from build123d import *

# Parameters (mm, degrees)
SKETCH_1_W          = 37.6
SKETCH_1_H          = 21
EXTRUDE_1_DEPTH     = 2
SKETCH_2_W          = 2.3
SKETCH_2_H          = 5.5
CUT_EXTRUDE_1_DEPTH = 22.626141588
SKETCH_4_W          = 13
SKETCH_4_H          = 10
EXTRUDE_2_DEPTH     = 2
EXTRUDE_4_DEPTH     = 10
SKETCH_6_R          = 6
CUT_EXTRUDE_2_DEPTH = 26.153329799
FILLET_1_R          = 2
FILLET_2_R          = 1


with BuildPart() as part:
    # 草图1 → 凸台-拉伸1 (new body)
    with BuildSketch(Plane.XY):
        Rectangle(SKETCH_1_W, SKETCH_1_H)
    extrude(amount=EXTRUDE_1_DEPTH)

    # 草图2 → 切除-拉伸1 (cut, through all)
    with BuildSketch(Plane.XY.offset(2)):
        with Locations((-17.65, 7.75)):
            Rectangle(SKETCH_2_W, SKETCH_2_H)
        with Locations((17.65, 7.75)):
            Rectangle(SKETCH_2_W, SKETCH_2_H)
        with Locations((-17.65, -7.75)):
            Rectangle(SKETCH_2_W, SKETCH_2_H)
        with Locations((17.65, -7.75)):
            Rectangle(SKETCH_2_W, SKETCH_2_H)
    extrude(amount=-CUT_EXTRUDE_1_DEPTH, mode=Mode.SUBTRACT)

    # 草图4 → 凸台-拉伸2 (add)
    with BuildSketch(Plane.ZY.offset(18.8)):
        with Locations((6.5, 0)):
            Rectangle(SKETCH_4_W, SKETCH_4_H)
    extrude_2 = extrude(amount=-EXTRUDE_2_DEPTH)

    # 草图5 → 凸台-拉伸4 (add)
    with BuildSketch(Plane(origin=(0, 5, 0), x_dir=(1, 0, 0), z_dir=(0, 1, 0))):
        Polygon((-8.740415593, -6.037395696), (-16.8, -10.690598923), (-16.8, -13), (-7.740415593, -7.769446504), align=None)
    extrude_4 = extrude(amount=-EXTRUDE_4_DEPTH)

    # 草图6 → 切除-拉伸2 (cut, through all)
    with BuildSketch(Plane(origin=(0, 0, 0), x_dir=(-1, 0, 0), z_dir=(0, 0, -1))):
        Circle(SKETCH_6_R)
    extrude(amount=-CUT_EXTRUDE_2_DEPTH, mode=Mode.SUBTRACT)

    # 镜向2: 凸台-拉伸2 across plane
    add(extrude_2.mirror(Plane(origin=(0, 0, 0), x_dir=(0, 0, 1), z_dir=(1, 0, 0))))

    # 镜向3: 凸台-拉伸4 across plane
    add(extrude_4.mirror(Plane(origin=(0, 0, 0), x_dir=(0, 0, 1), z_dir=(1, 0, 0))))

    # 圆角1
    fillet_1_edges = [part.edges().sort_by_distance(p)[0] for p in [
        (18.8, 0, 13),
        (-18.8, 0, 13),
    ]]
    fillet(fillet_1_edges, radius=FILLET_1_R - 0.0001)  # a hair under: the kernel refuses the full size

    # 圆角2
    fillet_2_edges = [part.edges().sort_by_distance(p)[0] for p in [
        (-18.8, 0, 0),
        (18.8, 0, 0),
    ]]
    fillet(fillet_2_edges, radius=FILLET_2_R)


solid = part.part
Design review of the part built by this model. Coordinates are the model's own, in mm. A direction names the side the tool comes from. Coordinates: 2 decimals unless noted, no trailing zeros. Order: outer loops, then holes, each group sorted by start corner. A loop starts at its lowest first (then second) coordinate and runs counter-clockwise, first axis right, second up. Notation, with made-up numbers: (66.5, 68.5) - (74.5, 68.5) arc R30 ccw to (74.5, 106.5) - close; hole circle Ø2 at (26.5, 19). An arc over 180 degrees is marked (long way). Put each result on its own line as item: value.
1) Wall thickness on L1, parallel to Y at x = 0, z = 0.85; L2, parallel to Z at x = -6, y = 2.75; L3, parallel to X at y = 3.25, z = 10: over which ranges is each line inside the solid? List them lowest first. Write a range as from..to.
Response values:
L1: y = -10.5..-6, 6..10.5
L2: z = 0..2
L3: x = -18.8..-16.8, -15.6..-11.6, 11.6..15.6, 16.8..18.8
2) The part is to be moulded in two halves that separate along Y. For faces 5 (the face through (6, 0, 1)), 6 (the face through (17, 5, 7)), 7 (the face through (17, -5, 7)), say which applies: released by +Y, released by -Y, zero draft, split by the parting line, or undercut.
Response values:
face 5: undercut
face 6: released by +Y
face 7: released by -Y
3) Take a section at A-A, the plane z = 3.5. Give the boundary of the cut face in (x, y), and give its area (3 significant figures).
Response values:
outline: (-18.8, -5) - (-16.8, -5) - (-16.8, 5) - (-18.8, 5) - close; (16.8, -5) - (18.8, -5) - (18.8, 5) - (16.8, 5) - close
area: 40.0 mm²
4) Take a section at D-D, the plane z = 9.5. Give the boundary of the cut face in (x, y).
Response values:
outline: (-18.8, -5) - (-16.8, -5) - (-16.8, 5) - (-18.8, 5) - close; (-14.74, -5) - (-10.74, -5) - (-10.74, 5) - (-14.74, 5) - close; (10.74, -5) - (14.74, -5) - (14.74, 5) - (10.74, 5) - close; (16.8, -5) - (18.8, -5) - (18.8, 5) - (16.8, 5) - close
5) Take a section at B-B, the plane x = 0. Give the boundary of the cut face in (y, z), and give its area (3 significant figures).
Response values:
outline: (-10.5, 0) - (-6, 0) - (-6, 2) - (-10.5, 2) - close; (6, 0) - (10.5, 0) - (10.5, 2) - (6, 2) - close
area: 18.0 mm²
6) Tool access review of faces 1 (the face through (-16.5, -8, 1)), 2 (the face through (-16.8, 0, 6)), 3 (the face through (12.3, 0.1, 10.4)), 4 (the face through (16.5, -8, 1)): name each direction out of +Z, -Z, +X, -X, +Y, -Y from which nothing blocks a thin tool from reaching the whole face with its end or side.
Response values:
face 1: +Z, -Z, -X, -Y
face 2: +Y, -Y
face 3: +Z, +Y, -Y
face 4: +Z, -Z, +X, -Y
7) Insertion check: P1, Ø6.5, axis at x = 3, y = 4, coming from the +Z side; P2, Ø0.6, axis at y = 7, z = 1, coming from the -X side; P3, Ø2, axis at y = 8, z = 1.5, coming from the +X side. Each pin has a flat end and moves straight along its axis. Give the tip position at first contact, or say it passes through.
Response values:
P1: stops at z = 2
P2: stops at x = -16.5
P3: stops at x = 16.5
